Model file for the job. Use its own axes, mm. Face numbers are marked on the shaded views. Round coordinates to 2 decimals unless told otherwise and drop trailing zeros. Order: outer loops, then holes, each group sorted by start corner. A loop starts at its lowest first (then second) coordinate and runs counter-clockwise, first axis right, second up. Notation, with made-up numbers: (-26, 43.25) - (28, 43.25) arc R5 cw to (28, 51.25) - close; hole circle Ø1 at (-28.5, 77). An arc over 180 degrees is marked (long way). Put each result on its own line as item: value. Start each with the question number.
Item 1: Saw through at C-C on y = 40. List the corners of the cut face in (x, z).
Item 2: Saw through at A-A on x = 2.5. List the corners of the cut face in (y, z), plus the area to 3 significant figures.
Item 3: Mould opens along Y. For the marked faces 1 and 2 say: pulls with the +Y half, pulls with the -Y half, needs draft (parallel to the pull), parting line crosses it, or undercut.
Item 4: Saw through at D-D on x = 88. List the corners of the cut face in (y, z).
Item 5: Saw through at B-B on y = 52.44. List the corners of the cut face in (x, z), plus the area to 3 significant figures.
Item 6: Pin check, flat tips, straight feed: pin 1 Ø1.2 at (y, z) = (24.5, 2.5) entering from +X; pin 2 Ø1 at (x, y) = (88.5, 11.5) entering from +Z; pin 3 Ø1.2 at (y, z) = (22, 3.5) entering from -X. Stop position of each tip, or through.
Item 7: Probe probe 1 along Y at (x, z) = (98, 0.4); probe 2 along X at (y, z) = (2.5, 0.55); probe 3 along X at (y, z) = (13.5, 4.8). List the from-to ranges inside material, lowest first.
Autodesk Inventor part; units mm, degrees
ref_plane "YZ Plane" through (0, 0, 0) normal (1, 0, 0) x (0, 1, 0)
ref_plane "XZ Plane" through (0, 0, 0) normal (0, 1, 0) x (-1, 0, 0)
ref_plane "XY Plane" through (0, 0, 0) normal (0, 0, 1) x (1, 0, 0)
sketch "Эскиз1" plane through (0, 0, 0) normal (0, 0, 1) x (1, 0, 0)
  line L0 (0, 0) -> (100.5, 0)
  line L1 (100.5, 0) -> (100.5, 54.94)
  line L2 (100.5, 54.94) -> (0, 54.94)
  line L3 (0, 54.94) -> (0, 0)
  circle A0 centre (2.5, 52.44) radius 1.5
  circle A1 centre (98, 52.44) radius 1.5
  line L4 (196, 54.94) -> (95.5, 54.94)
  circle A2 centre (2.5, 2.5) radius 1.5
  circle A3 centre (98, 2.5) radius 1.5
  dimension "d0" = 100.5
  dimension "d1" = 54.94
  dimension "d2" = 3
  dimension "d3" = 2.5
  dimension "d4" = 2.5
  dimension "d7" = 95.5
  dimension "d14" = 49.94
extrude "Выдавливание1" add sketch "Эскиз1" along normal blind 5.45
sketch "Эскиз2" plane through (0, 0, 5.45) normal (0, 0, 1) x (1, 0, 0)
  line L0 (9, 54.94) -> (94.5, 54.94)
  line L1 (94.5, 54.94) -> (94.5, 0)
  line L2 (94.5, 0) -> (9, 0)
  line L3 (9, 0) -> (9, 54.94)
  line L4 (100.5, 54.94) -> (0, 54.94)
  line L5 (100.5, 0) -> (100.5, 54.94)
  line L6 (-12, 65) -> (119, 65)
  line L7 (119, 65) -> (119, -14)
  line L8 (119, -14) -> (-12, -14)
  line L9 (-12, -14) -> (-12, 65)
  point P0 (0, 0)
  point P1 (50.25, 54.94)
  dimension "d21" = 85.5
  dimension "d22" = 54.94
  dimension "d23" = 6
extrude "Выдавливание2" cut sketch "Эскиз2" against normal blind 4.1
sketch "Эскиз3" plane through (0, 0, 5.45) normal (0, 0, 1) x (1, 0, 0)
  line L0 (10, 53.94) -> (89.5, 53.94)
  line L1 (89.5, 53.94) -> (89.5, 1)
  line L2 (89.5, 1) -> (10, 1)
  line L3 (10, 1) -> (10, 53.94)
  line L4 (94.5, 54.94) -> (9, 54.94)
  line L5 (9, 54.94) -> (9, 0)
  line L6 (9, 0) -> (94.5, 0)
  line L7 (94.5, 0) -> (94.5, 54.94)
  point P0 (0, 0)
  dimension "d28" = 1
  dimension "d29" = 1
  dimension "d30" = 1
  dimension "d31" = 5
extrude "Выдавливание3" cut sketch "Эскиз3" against normal blind 1 contours L0 L1 L2 L3
properties part number "NextionDisplay"
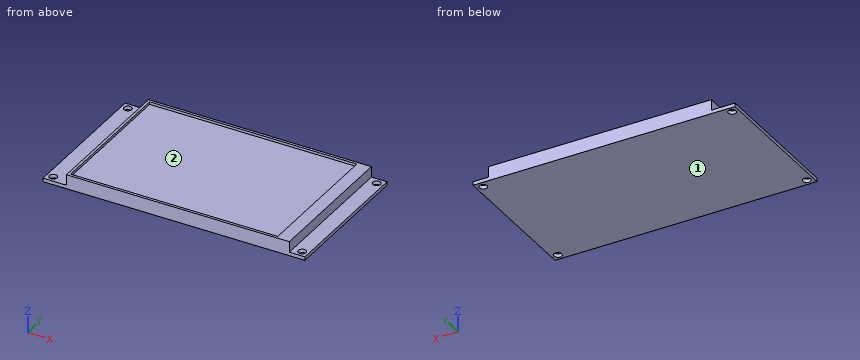
Results found:
1. outline: (0, 0) - (100.5, 0) - (100.5, 1.35) - (94.5, 1.35) - (94.5, 5.45) - (89.5, 5.45) - (89.5, 4.45) - (10, 4.45) - (10, 5.45) - (9, 5.45) - (9, 1.35) - (0, 1.35) - close
2. outline: (0, 0) - (1, 0) - (1, 1.35) - (0, 1.35) - close; (4, 0) - (50.94, 0) - (50.94, 1.35) - (4, 1.35) - close; (53.94, 0) - (54.94, 0) - (54.94, 1.35) - (53.94, 1.35) - close
2. area: 66.1 mm²
3. face 1: needs draft
3. face 2: undercut
4. outline: (0, 0) - (54.94, 0) - (54.94, 5.45) - (53.94, 5.45) - (53.94, 4.45) - (1, 4.45) - (1, 5.45) - (0, 5.45) - close
5. outline: (0, 0) - (1, 0) - (1, 1.35) - (0, 1.35) - close; (4, 0) - (96.5, 0) - (96.5, 1.35) - (94.5, 1.35) - (94.5, 5.45) - (89.5, 5.45) - (89.5, 4.45) - (10, 4.45) - (10, 5.45) - (9, 5.45) - (9, 1.35) - (4, 1.35) - close; (99.5, 0) - (100.5, 0) - (100.5, 1.35) - (99.5, 1.35) - close
5. area: 399 mm²
6. pin 1: stops at x = 94.5
6. pin 2: stops at z = 4.45
6. pin 3: stops at x = 9
7. probe 1: y = 0 to 1, 4 to 50.94, 53.94 to 54.94
7. probe 2: x = 0 to 1, 4 to 96.5, 99.5 to 100.5
7. probe 3: x = 9 to 10, 89.5 to 94.5
